The listing builds one solid part. Answer for the finished solid, in the listing's coordinates (mm). Give positions to 0.01 mm unless a question says otherwise; leave off trailing zeros. Write each loop counter-clockwise with the first axis right and the second up, starting at its lowest first coordinate (ties: lowest second). Pieces come first, ordered by that corner, then holes. Notation, with made-up numbers: M -23.75,72.25 L 22.25,72.25 A28 ccw 22.25,99.25 Z; hole C 84,7.5 d3. An arc over 180 degrees is marked long. Return JSON: item names as keys, results as strings.
Autodesk Inventor part; units mm, degrees
ref_plane "YZ Plane" through (0, 0, 0) normal (1, 0, 0) x (0, 1, 0)
ref_plane "XZ Plane" through (0, 0, 0) normal (0, 1, 0) x (-1, 0, 0)
ref_plane "XY Plane" through (0, 0, 0) normal (0, 0, 1) x (1, 0, 0)
sketch "Sketch1" plane through (0, 0, 0) normal (0, 0, 1) x (1, 0, 0)
  line L0 (-15.7, 12.7) -> (-12.7, 12.7)
  line L1 (-12.7, 12.7) -> (-12.7, -9.7)
  line L2 (-12.7, -9.7) -> (12.7, -9.7)
  line L3 (12.7, -9.7) -> (12.7, 12.7)
  line L4 (12.7, 12.7) -> (15.7, 12.7)
  line L5 (15.7, 12.7) -> (15.7, -12.7)
  line L6 (15.7, -12.7) -> (-15.7, -12.7)
  line L7 (-15.7, -12.7) -> (-15.7, 12.7)
  point P0 (0, 0)
  dimension "d0" = 3
  dimension "d2" = 3
  dimension "d3" = 25.4
  dimension "d4" = 31.4
  dimension "d5" = 15.7
  dimension "d7" = 12.7
  dimension "d8" = 3
extrude "Extrusion1" add sketch "Sketch1" against normal blind 457.2
sketch "Sketch7" plane through (-15.7, -12.7, 0) normal (0, -1, 0) x (1, 0, 0)
  circle A0 centre (13.8784, -447.9) radius 3.175
  point P0 (15.7, 0)
  dimension "d25" = 6.35
extrude "Extrusion5" cut sketch "Sketch7" against normal blind 10
sketch "Sketch8" plane through (-15.7, -12.7, 0) normal (0, -1, 0) x (1, 0, 0)
  line L0 (0, -184) -> (31.4, -184) construction
  line L1 (31.4, -134) -> (0, -134) construction
  line L2 (31.4, -134) -> (31.4, -184) construction
  line L3 (15.7, -134) -> (15.7, -159) construction
  line L4 (15.7, -159) -> (31.4, -159) construction
  circle A0 centre (15.7, -159) radius 3.175
  point P0 (15.7, 0)
  dimension "d29" = 6.35
extrude "Extrusion6" cut sketch "Sketch8" against normal blind 10
sketch "Sketch9" plane through (-15.7, -12.7, 0) normal (0, -1, 0) x (1, 0, 0)
  circle A0 centre (13.8784, -9.3) radius 3.175
  circle A1 centre (15.7, -29) radius 3.175
  point P0 (15.7, 0)
extrude "Extrusion7" cut sketch "Sketch9" against normal blind 10
equation "\"d2\" = d0"
equation "\"d8\" = d0"
properties part number "18in C-Channel Front" material "Aluminum 6061"
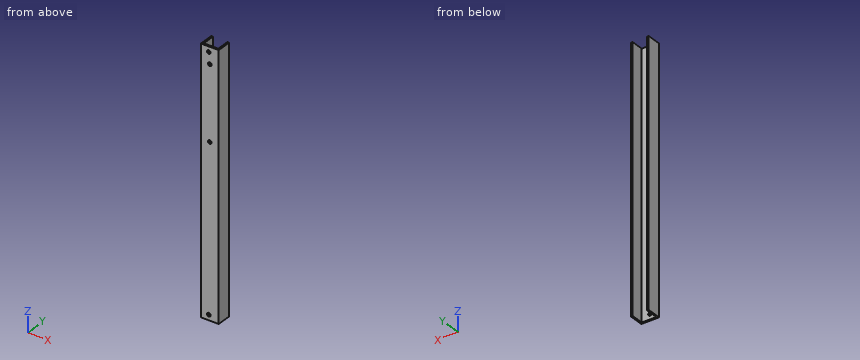
Item 1: A cutting plane is placed at A-A, the plane y = -0.5. Write down the section's boundary in (x, z), plus the area to 3 significant figures.
Geometry results:
{"outline": "M -15.7,-457.2 L -12.7,-457.2 L -12.7,0 L -15.7,0 Z; M 12.7,-457.2 L 15.7,-457.2 L 15.7,0 L 12.7,0 Z", "area": "2,740 mm2"}
Item 2: Given pin 1 Ø4 at (x, z) = (0, -29) entering from +Y; pin 2 Ø7.5 at (x, z) = (-4, -155) entering from +Y, each flat-ended and moving along its own axis, determine where each tip first touches the part or whether it passes through.
Geometry results:
{"pin 1": "passes through", "pin 2": "stops at y = -9.7"}
Item 3: Find the intervals of material crossed by line 1 (X direction, y = 11, z = -163); line 2 (Z direction, x = 0, y = -11.8) (3 decimals); line 3 (X direction, y = -11.2, z = -447.9), in increasing order.
Geometry results:
{"line 1": "x = -15.7 to -12.7, 12.7 to 15.7", "line 2": "z = -457.2 to -450.5, -445.3 to -162.175, -155.825 to -32.175, -25.825 to -11.9, -6.7 to 0", "line 3": "x = -15.7 to -5, 1.35 to 15.7"}
Item 4: A cutting plane is placed at B-B, the plane z = -222.5. Write down the section's boundary in (x, y).
Geometry results:
{"outline": "M -15.7,-12.7 L 15.7,-12.7 L 15.7,12.7 L 12.7,12.7 L 12.7,-9.7 L -12.7,-9.7 L -12.7,12.7 L -15.7,12.7 Z"}
